from build123d import *

# Parameters (mm, degrees)
ESQUISSE1_W             = 90
ESQUISSE1_H             = 15
BOSS_EXTRU_1_DEPTH      = 15
ESQUISSE2_W             = 13
ESQUISSE2_H             = 13
ENL_V_MAT_EXTRU_1_DEPTH = 92.549167118
D_GAGEMENT_M31_D        = 3.4
D_GAGEMENT_M31_DEPTH    = 24
D_GAGEMENT_M31_TIP      = 1.021463052
ESQUISSE5_W             = 40
ESQUISSE5_H             = 13
ENL_V_MAT_EXTRU_2_DEPTH = 50.183330509
D_GAGEMENT_M2_51_D      = 2.9
D_GAGEMENT_M2_51_DEPTH  = 24
D_GAGEMENT_M2_51_TIP    = 0.871247898


with BuildPart() as part:
    # Esquisse1 → Boss.-Extru.1 (new body)
    with BuildSketch(Plane(origin=(0, 0, 0), x_dir=(1, 0, 0), z_dir=(0, 1, 0))):
        Rectangle(ESQUISSE1_W, ESQUISSE1_H)
    extrude(amount=BOSS_EXTRU_1_DEPTH)

    # Esquisse2 → Enlèv. mat.-Extru.1 (cut, through all)
    with BuildSketch(Plane.ZY.offset(45)):
        with Locations((-1, 8.5)):
            Rectangle(ESQUISSE2_W, ESQUISSE2_H)
    extrude(amount=-ENL_V_MAT_EXTRU_1_DEPTH, mode=Mode.SUBTRACT)

    # Dégagement M31
    with Locations(Plane(origin=(0, 2, 0), x_dir=(1, 0, 0), z_dir=(0, 1, 0))):
        with Locations((-41.5, 0), (41.5, 0)):
            Hole(D_GAGEMENT_M31_D / 2, depth=D_GAGEMENT_M31_DEPTH)
            with Locations((0, 0, -(D_GAGEMENT_M31_DEPTH + D_GAGEMENT_M31_TIP / 2))):  # 118° drill point
                Cone(0, D_GAGEMENT_M31_D / 2, D_GAGEMENT_M31_TIP, mode=Mode.SUBTRACT)

    # Esquisse5 → Enlèv. mat.-Extru.2 (cut, through all)
    with BuildSketch(Plane(origin=(0, 0, 5.5), x_dir=(-1, 0, 0), z_dir=(0, 0, -1))):
        with Locations((25, 8.5)):
            Rectangle(ESQUISSE5_W, ESQUISSE5_H)
        with Locations((-25, 8.5)):
            Rectangle(ESQUISSE5_W, ESQUISSE5_H)
    extrude(amount=-ENL_V_MAT_EXTRU_2_DEPTH, mode=Mode.SUBTRACT)

    # Dégagement M2.51
    with Locations(Plane(origin=(0, 0, 5.5), x_dir=(-1, 0, 0), z_dir=(0, 0, -1))):
        with Locations((0, 4)):
            Hole(D_GAGEMENT_M2_51_D / 2, depth=D_GAGEMENT_M2_51_DEPTH)
            with Locations((0, 0, -(D_GAGEMENT_M2_51_DEPTH + D_GAGEMENT_M2_51_TIP / 2))):  # 118° drill point
                Cone(0, D_GAGEMENT_M2_51_D / 2, D_GAGEMENT_M2_51_TIP, mode=Mode.SUBTRACT)


solid = part.part
Source: CAD feature listing. Evaluate the final solid. Frame: model axes, mm. A direction names the side the tool comes from. Give positions to 0.01 mm unless a question says otherwise; leave off trailing zeros. Write each loop counter-clockwise with the first axis right and the second up, starting at its lowest first coordinate (ties: lowest second). Pieces come first, ordered by that corner, then holes. Notation, with made-up numbers: (80.25, 2) -> (122.25, 2) arc R24 ccw to (122.25, 14) -> close; hole circle Ø4 at (-5, -20). An arc over 180 degrees is marked (long way). Return JSON: item names as keys, results as strings. Group by question number.
1. Mould query, pull axis X, two halves, no side actions, for faces 1 (the face through (-40.15, 0.99, 1.03)), 2 (the face through (0, 8, 5.5)), 3 (the face through (45, 1, 0)). Classes: +X half, -X half, draft (parallel to the pull), parting line (faces both ways), or undercut.
2. Access query for faces 4 (the face through (5, 8, 6)), 5 (the face through (-5, 8, 6)), 6 (the face through (-45, 1, 0)). Directions: +Z, -Z, +X, -X, +Y, -Y. A direction counts if a zero-diameter tool reaches every point of the face in a straight line with its end or side. Return the directions, or none.
3. Material intervals for line 1 (Z direction, x = -41.5, y = 1.45); line 2 (Y direction, x = 0, z = 7.15); line 3 (Y direction, x = -26, z = 2.5), sorted ascending. Write a range as from..to.
4. Section D-D, the plane x = -41.5. Output: boundary loops of the cut face in (y, z).
5. Section A-A, the plane z = 0. Output: boundary loops of the cut face in (x, y), then the cut area to 3 significant figures.
6. Section B-B, the plane x = 0. Output: boundary loops of the cut face in (y, z), then the cut area to 3 significant figures.
7. Section C-C, the plane y = 4. Output: boundary loops of the cut face in (x, z), then the cut area to 3 significant figures.
8. Pin query (flat end, axial travel): pin 1 Ø1.6 at (y, z) = (7.5, 7) entering from -X; pin 2 Ø0.6 at (y, z) = (8.5, 6) entering from +X; pin 3 Ø5 at (x, z) = (16, -5) entering from +Y; pin 4 Ø4.5 at (x, y) = (0, 4) entering from -Z. Return the tip coordinate at first contact, or that it passes through.
Determined:
{
 "1": {"face 1": "undercut", "face 2": "draft", "face 3": "+X half"},
 "2": {"face 4": "+Z, -Z, +X, +Y", "face 5": "+Z, -Z, -X, +Y", "face 6": "+Z, -Z, -X, +Y, -Y"},
 "3": {"line 1": "z = -7.5..-1.7, 1.7..7.5", "line 2": "y = 0..2.55, 5.45..15", "line 3": "y = 0..2"},
 "4": {"outline": "(0, -7.5) -> (2, -7.5) -> (2, -1.7) -> (0, -1.7) -> close; (0, 1.7) -> (2, 1.7) -> (2, 7.5) -> (0, 7.5) -> close"},
 "5": {"outline": "(-45, 0) -> (-43.2, 0) -> (-43.2, 2) -> (-45, 2) -> close; (-39.8, 0) -> (39.8, 0) -> (39.8, 2) -> (-39.8, 2) -> close; (43.2, 0) -> (45, 0) -> (45, 2) -> (43.2, 2) -> close", "area": "166 mm2"},
 "6": {"outline": "(0, -7.5) -> (2, -7.5) -> (2, 5.5) -> (2.55, 5.5) -> (2.55, 7.5) -> (0, 7.5) -> close; (5.45, 5.5) -> (15, 5.5) -> (15, 7.5) -> (5.45, 7.5) -> close", "area": "50.2 mm2"},
 "7": {"outline": "(-5, 5.5) -> (-1.45, 5.5) -> (-1.45, 7.5) -> (-5, 7.5) -> close; (1.45, 5.5) -> (5, 5.5) -> (5, 7.5) -> (1.45, 7.5) -> close", "area": "14.2 mm2"},
 "8": {"pin 1": "stops at x = -5", "pin 2": "stops at x = 5", "pin 3": "stops at y = 2", "pin 4": "stops at z = -7.5"}
}
